Verification items for the finished model (mm, model axes). Coordinates: 2 decimals unless noted, no trailing zeros. Order: outer loops, then holes, each group sorted by start corner. A loop starts at its lowest first (then second) coordinate and runs counter-clockwise, first axis right, second up.
Q1. Cross-section at A-A, the plane z = 163.5. Record the boundary of the cut face in (x, y).
Q2. Thickness scan on line 1 (Z direction, x = 35, y = -341); line 2 (Y direction, x = 26, z = 279.5); line 3 (Z direction, x = 28, y = -166). Record the ranges inside material, lowest first.
Q3. Depth check by flat-ended pin: P1, Ø14, axis at y = -329.4, z = -56.85, coming from the +X side; P2, Ø9, axis at x = 9.5, y = 106, coming from the +Z side; P3, Ø5, axis at x = 10.5, z = 25, coming from the +Y side. Enter the tip coordinate at first touch or a pass-through.
Q4. Cross-section at B-B, the plane y = -219.5. Record the boundary of the cut face in (x, z).
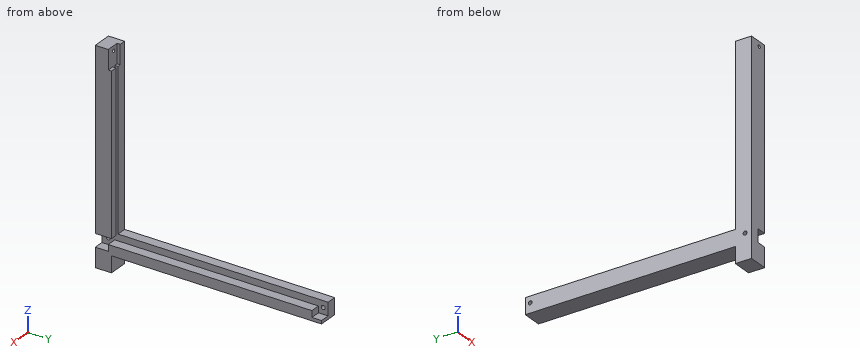
from build123d import *

# Parameters (mm, degrees)
F1_DEPTH = 60
F3_DEPTH = 30
F5_D     = 12
F7_DEPTH = 10
F9_D     = 10


with BuildPart() as f1:
    # F0 (on Right) → F1 (new body)
    with BuildSketch(Plane.YZ):
        Polygon((-299.395279, -136.848614), (-299.395279, -86.848614), (350.604721, -86.848614), (350.604721, -36.848614), (-299.395279, -36.848614), (-299.395279, 513.151386), (-349.395279, 513.151386), (-349.395279, -36.848614), (-349.395279, -86.848614), (-349.395279, -136.848614), align=None)
    extrude(amount=F1_DEPTH)

    # F2 (on face) → F3 (cut)
    with BuildSketch(Plane.YZ.offset(60)):
        Polygon((-309.395279, -36.848614), (-349.395279, -36.848614), (-349.395279, -76.848614), (-309.395279, -76.848614), (-309.395279, -56.848614), (320.604721, -56.848614), (320.604721, -76.848614), (350.604721, -76.848614), (350.604721, -36.848614), align=None)
    extrude(amount=-F3_DEPTH, mode=Mode.SUBTRACT)

    # F5 (through all)
    with Locations(Plane.YZ.offset(30)):
        with Locations((-329.395279, -56.848614), (335.604721, -56.848614)):
            Hole(F5_D / 2)

    # F6 (on face) → F7 (cut)
    with BuildSketch(Plane(origin=(0, -299.395279, 0), x_dir=(-1, 0, 0), z_dir=(0, 1, 0))):
        Polygon((-40, -36.848614), (-30, -36.848614), (-30, 453.151386), (-20, 453.151386), (-20, 513.151386), (-60, 513.151386), (-60, 463.151386), (-60, 453.151386), (-40, 453.151386), align=None)
    extrude(amount=-F7_DEPTH, mode=Mode.SUBTRACT)

    # F9 (through all)
    with Locations(Plane(origin=(0, -309.395279, 0), x_dir=(-1, 0, 0), z_dir=(0, 1, 0))):
        with Locations((-35, 498.151386)):
            Hole(F9_D / 2)


solid = f1.part
Check values:
1. outline: (0, -349.4) - (60, -349.4) - (60, -299.4) - (40, -299.4) - (40, -309.4) - (30, -309.4) - (30, -299.4) - (0, -299.4) - close
2. line 1: z = -136.85 to -76.85, -36.85 to 493.15, 503.15 to 513.15
2. line 2: y = -349.4 to -299.4
2. line 3: z = -86.85 to -36.85
3. P1: stops at x = 30
3. P2: stops at z = -36.85
3. P3: stops at y = -299.4
4. outline: (0, -86.85) - (60, -86.85) - (60, -56.85) - (30, -56.85) - (30, -36.85) - (0, -36.85) - close
